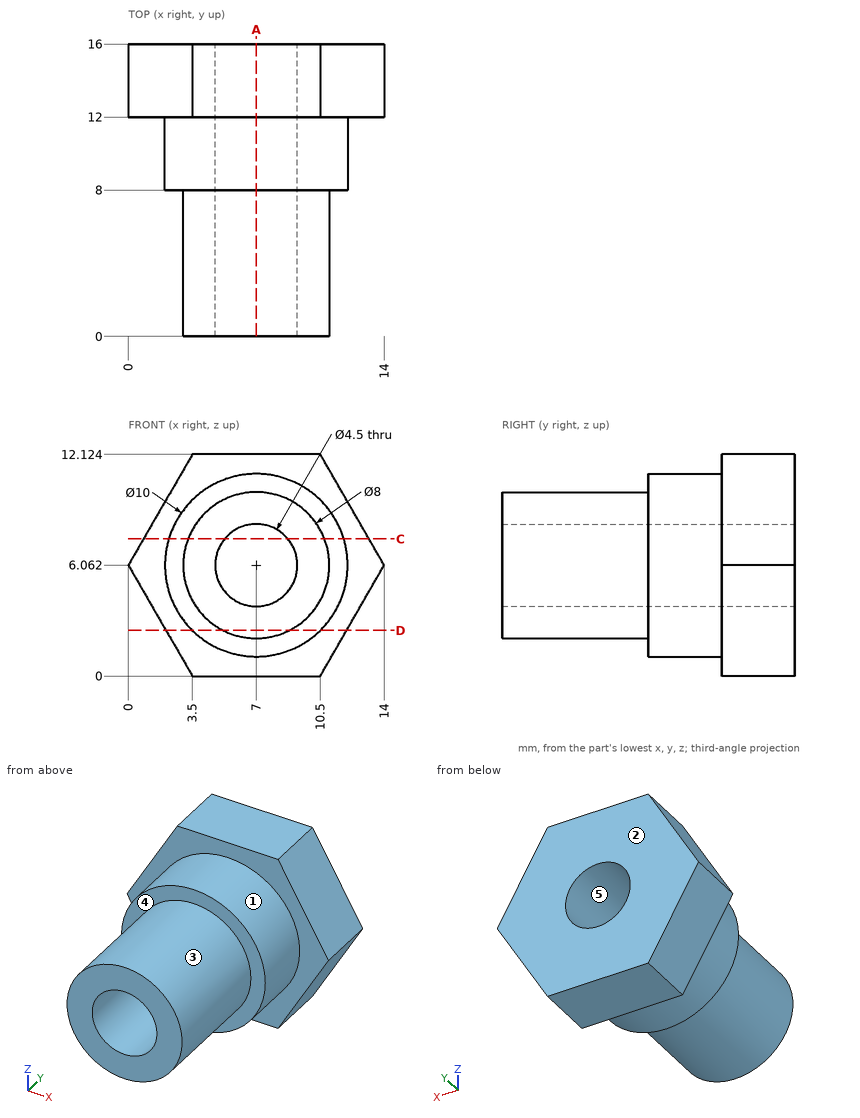
Here's the drawing with two shaded views (mm, measured from the low corner). I have some questions. A direction names the side the tool comes from. Round coordinates to 2 decimals unless told otherwise and drop trailing zeros. Loops run counter-clockwise (first coordinate to the right, second up) from the corner with the lowest first, then second, coordinate; pieces in that order, holes last.
1. Suppose I cut it at A-A, the plane x = 7. Please give me the cut outline in (y, z) (1 decimal).
Answers:
outline: (0, 2.1) - (8, 2.1) - (8, 1.1) - (12, 1.1) - (12, 0) - (16, 0) - (16, 3.8) - (0, 3.8) - close; (0, 8.3) - (16, 8.3) - (16, 12.1) - (12, 12.1) - (12, 11.1) - (8, 11.1) - (8, 10.1) - (0, 10.1) - close
2. Suppose I cut it at C-C, the plane z = 7.5. Please give me the cut outline in (x, y).
Answers:
outline: (0.83, 12) - (2.21, 12) - (2.21, 8) - (3.27, 8) - (3.27, 0) - (5.27, 0) - (5.27, 16) - (0.83, 16) - close; (8.73, 0) - (10.73, 0) - (10.73, 8) - (11.79, 8) - (11.79, 12) - (13.17, 12) - (13.17, 16) - (8.73, 16) - close
3. Thinking about a two-plate mould opening in X: for the marked faces 3, 4 and 5, which applies, released by +X, released by -X, zero draft, split by the parting line, or undercut?
Answers:
face 3: split by the parting line
face 4: zero draft
face 5: undercut
4. Suppose I cut it at D-D, the plane z = 2.5. Please give me the cut outline in (x, y).
Answers:
outline: (2.06, 12) - (3.49, 12) - (3.49, 8) - (5.18, 8) - (5.18, 0) - (8.82, 0) - (8.82, 8) - (10.51, 8) - (10.51, 12) - (11.94, 12) - (11.94, 16) - (2.06, 16) - close
5. For the marked faces 1 and 2, which set-ups out of +Z, -Z, +X, -X, +Y, -Y let a thin tool reach every point of the face, with its end or its side?
Answers:
face 1: -Y
face 2: +Z, -Z, +X, -X, +Y
6. Will these pins go through, and if not, where does the flat tip stop? pin 1 (1 mm diameter, centred on x = 4, y = 4, fed in from -Z); pin 2 (1 mm diameter, centred on x = 9, y = 10, fed in from -Z); pin 3 (1 mm diameter, centred on y = 7, z = 7, fed in from -X).
Answers:
pin 1: stops at z = 2.94
pin 2: stops at z = 1.29
pin 3: stops at x = 3.02
7. If I drill on probe 1 along Z at (x, y) = (7, 5); probe 2 along Z at (x, y) = (7, 10.5); probe 3 along Y at (x, z) = (11, 7.25), over which ranges is the centre line in solid material (lowest first)?
Answers:
probe 1: z = 2.06 to 3.81, 8.31 to 10.06
probe 2: z = 1.06 to 3.81, 8.31 to 11.06
probe 3: y = 8 to 16
